Study the drawing (mm; zero at the part's minimum x, y, z) and answer. A direction names the side the tool comes from. Coordinates: 2 decimals unless noted, no trailing zeros. Loops run counter-clockwise (first coordinate to the right, second up) from the corner with the lowest first, then second, coordinate; pieces in that order, holes last. Notation, with made-up numbers: (88, 74) - (105, 74) arc R21 ccw to (105, 95) - close; hole circle Ø4 at (86.5, 46.5). An arc over 180 degrees is marked (long way). Use one line per item in the form item = value. Start each with the question number.
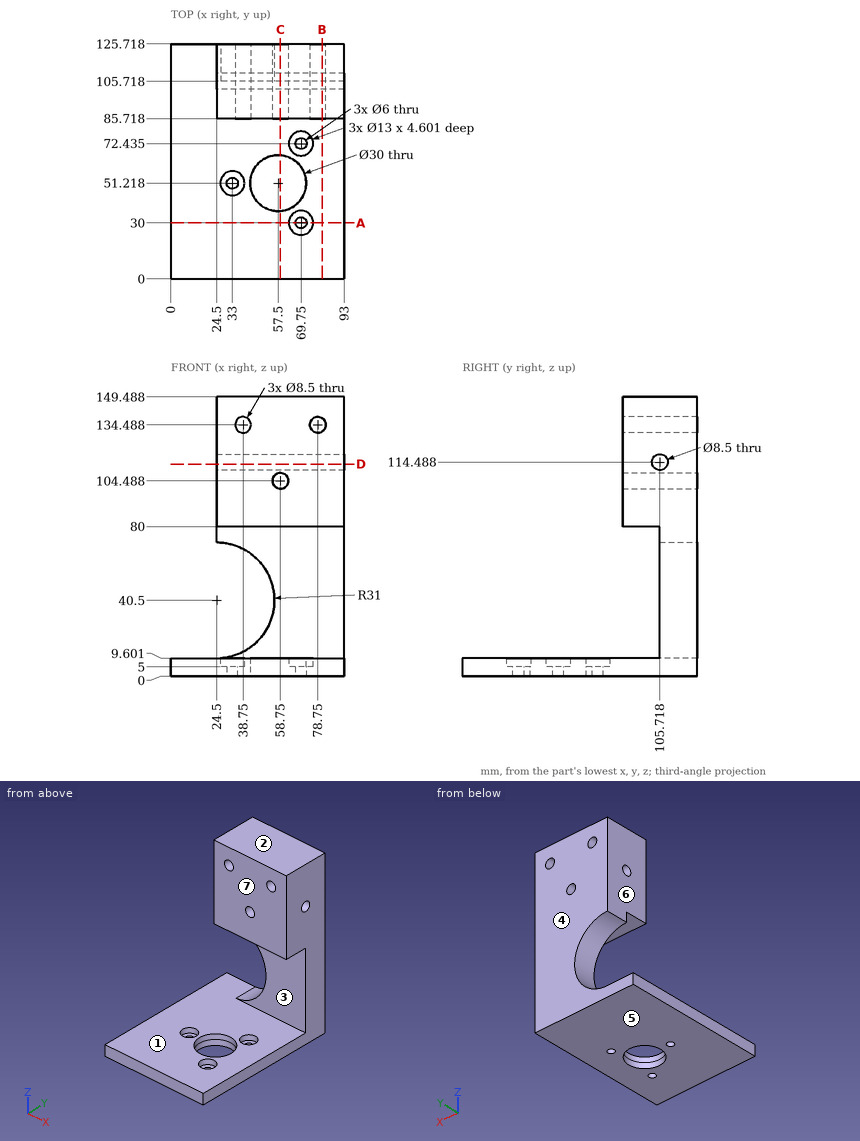
(1) A cutting plane is placed at C-C (x = 58.75). State how many separate pieces and enclosed holes the cut face has, then the cut area to 3 significant figures.
(2) Each of these flat-tipped pins is pushed along its axis until it touches: pin 1 Ø20.5 at (x, z) = (48.5, 99) entering from -Y; pin 2 Ø20 at (y, z) = (101.5, 92.5) entering from -X; pin 3 Ø6.5 at (x, y) = (68, 27.5) entering from +Z; pin 4 Ø7.5 at (x, z) = (58.75, 104.488) entering from -Y. Where does it stop, or does it pass through?
(3) Find the intervals of material crossed by probe 1 along Z at (x, y) = (78.75, 95); probe 2 along Z at (x, y) = (58.75, 111.5); probe 3 along Z at (x, y) = (61, 97) (1 decimal), in increasing order. Write a range as from..to.
(4) For the marked faces 5, 6 and 7, determine the directions among +Z, -Z, +X, -X, +Y, -Y from which every point of the face is accessible in a straight line to the end or side of a thin tool.
(5) Determine the mould class of the marked faces 1, 2, 3 and 4 for opening direction Z: +Z half, -Z half, draft (parallel to the pull), parting line (faces both ways), or undercut.
(6) A cutting plane is placed at B-B (x = 81). Determine the outline of the cut face in (y, z), then the cut area to 3 significant figures.
(7) A cutting plane is placed at D-D (z = 113.5). Determine the outline of the cut face in (x, y), then the cut area to 3 significant figures.
(8) A cutting plane is placed at A-A (y = 30). Determine the outline of the cut face in (x, z), then the cut area to 3 significant figures.
Evaluation:
q1.separate_pieces = 3
q1.enclosed_holes = 1
q1.area = 4,710 mm^2
q2.pin_1 = 85.72
q2.pin_2 = 24.5
q2.pin_3 = 5
q2.pin_4 = through
q3.probe_1 = 0..9.6, 80..130.24, 138.74..149.49
q3.probe_2 = 0..100.24, 108.74..149.49
q3.probe_3 = 0..9.6, 80..100.9, 108.1..149.5
q4.face_5 = -Z, +X, -X, +Y, -Y
q4.face_6 = +Z, -X, +Y, -Y
q4.face_7 = +Z, +X, -X, -Y
q5.face_1 = undercut
q5.face_2 = +Z half
q5.face_3 = undercut
q5.face_4 = draft
q6.outline = (0, 0) - (125.72, 0) - (125.72, 130.88) - (85.72, 130.88) - (85.72, 80) - (105.72, 80) - (105.72, 9.6) - (0, 9.6) - close; (85.72, 138.09) - (125.72, 138.09) - (125.72, 149.49) - (85.72, 149.49) - close; hole circle Ø8.5 at (105.72, 114.49)
q6.area = 5,050 mm^2
q7.outline = (24.5, 85.72) - (93, 85.72) - (93, 101.58) - (24.5, 101.58) - close; (24.5, 109.85) - (93, 109.85) - (93, 125.72) - (24.5, 125.72) - close
q7.area = 2,170 mm^2
q8.outline = (0, 0) - (66.75, 0) - (66.75, 5) - (63.25, 5) - (63.25, 9.6) - (0, 9.6) - close; (72.75, 0) - (93, 0) - (93, 9.6) - (76.25, 9.6) - (76.25, 5) - (72.75, 5) - close
q8.area = 803 mm^2
